Verification items for the finished model (mm, model axes). Face numbers are marked on the shaded views. A direction names the side the tool comes from. Round coordinates to 2 decimals unless told otherwise and drop trailing zeros. Order: outer loops, then holes, each group sorted by start corner. A loop starts at its lowest first (then second) coordinate and runs counter-clockwise, first axis right, second up. Notation, with made-up numbers: M 5,63.25 L 56,63.25 A6 cw 56,70.25 Z; hole C 85,-34.75 d10. An arc over 180 degrees is marked long. Answer as a JSON object with one key per item and string values. Group by question number.
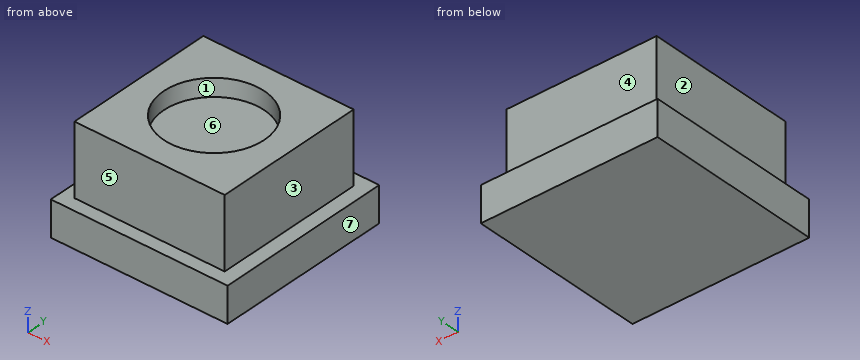
```python
from build123d import *

# Parameters (mm, degrees)
F0_W     = 25.4
F0_H     = 25.4
F0_W_2   = 21.59
F0_H_2   = 21.59
F1_DEPTH = 5.08
F0_R     = 7.215884
F2_DEPTH = 15.24
F3_DEPTH = 12.7


with BuildPart() as f1:
    # F0 (on Top) → F1 (new body)
    with BuildSketch(Plane.XY):
        with Locations((-38.394353, 12.483482)):
            Rectangle(F0_W, F0_H)
        with Locations((-38.49318, 12.438105)):
            Rectangle(F0_W_2, F0_H_2, mode=Mode.SUBTRACT)
    extrude(amount=F1_DEPTH)

    # F0 (on Top) → F2 (join)
    with BuildSketch(Plane.XY):
        with Locations((-38.49318, 12.438105)):
            Rectangle(F0_W_2, F0_H_2)
        with Locations((-38.49318, 12.438105)):
            Circle(F0_R, mode=Mode.SUBTRACT)
    extrude(amount=F2_DEPTH)

    # F0 (on Top) → F3 (join)
    with BuildSketch(Plane.XY):
        with Locations((-38.49318, 12.438105)):
            Circle(F0_R)
    extrude(amount=F3_DEPTH)


solid = f1.part
```
Q1. Cross-section at C-C, the plane z = 6.5. Record the cut outline in (x, y).
Q2. Tool access check on the marked faces 1, 2, 3 and 4. Record the directions out of +Z, -Z, +X, -X, +Y, -Y that give a thin tool (end or side, any length) a straight path to the whole face; none if there is none.
Q3. Gauge pin test, flat ends, axial feed: pin 1 Ø3 at (x, y) = (-35, 9.5) entering from +Z; pin 2 Ø5 at (y, z) = (8, 9) entering from -X; pin 3 Ø8 at (x, z) = (-35, 10.5) entering from -Y. Record the tip position at first contact, or that the pin passes through.
Q4. Cross-section at B-B, the plane x = -48.5. Record the cut outline in (y, z).
Q5. Thickness scan on line 1 (Y direction, x = -41.25, z = 8); line 2 (X direction, y = 4.25, z = 13); line 3 (Z direction, x = -42.25, y = 9.25). Record the ranges inside material, lowest first. Write a range as from..to.
Q6. Release check for a two-part mould opening along Y. For the marked faces 5, 6 and 7 record: released by +Y, released by -Y, zero draft, split by the parting line, or undercut.
Q7. Cross-section at A-A, the plane y = 20.5. Record the cut outline in (x, z), then the cut area to 3 significant figures.
Q8. Cross-section at D-D, the plane x = -42. Record the cut outline in (y, z).
Conclusion:
{
 "1": {"outline": "M -49.29,1.64 L -27.7,1.64 L -27.7,23.23 L -49.29,23.23 Z"},
 "2": {"face 1": "+Z", "face 2": "+Z, -X, +Y, -Y", "face 3": "+Z, +X, +Y, -Y", "face 4": "+Z, +X, -X, +Y"},
 "3": {"pin 1": "z = 12.7", "pin 2": "x = -49.29", "pin 3": "y = 1.64"},
 "4": {"outline": "M -0.22,0 L 25.18,0 L 25.18,5.08 L 23.23,5.08 L 23.23,15.24 L 1.64,15.24 L 1.64,5.08 L -0.22,5.08 Z"},
 "5": {"line 1": "1.64..23.23", "line 2": "-49.29..-27.7", "line 3": "0..12.7"},
 "6": {"face 5": "released by -Y", "face 6": "undercut", "face 7": "zero draft"},
 "7": {"outline": "M -51.09,0 L -25.69,0 L -25.69,5.08 L -27.7,5.08 L -27.7,15.24 L -49.29,15.24 L -49.29,5.08 L -51.09,5.08 Z", "area": "348 mm2"},
 "8": {"outline": "M -0.22,0 L 25.18,0 L 25.18,5.08 L 23.23,5.08 L 23.23,15.24 L 18.74,15.24 L 18.74,12.7 L 6.13,12.7 L 6.13,15.24 L 1.64,15.24 L 1.64,5.08 L -0.22,5.08 Z"}
}
